Can you work these out from the model? Positions are in its coordinate system, mm. A direction names the side the tool comes from. Give positions to 0.01 mm unless a question says otherwise; leave off trailing zeros. Loops run counter-clockwise (first coordinate to the right, second up) from the corner with the lowest first, then second, coordinate; pieces in that order, holes last.
from build123d import *

# Parameters (mm, degrees)
BOSS_EXTRUDE1_DEPTH = 1.5
SKETCH2_R           = 3.38382201
BOSS_EXTRUDE2_DEPTH = 4.5
SKETCH3_R           = 2.5
CUT_EXTRUDE1_DEPTH  = 3
SKETCH4_R           = 1
CUT_EXTRUDE2_DEPTH  = 3.5
SKETCH5_R           = 0.55
CUT_EXTRUDE3_DEPTH  = 3.5
SCALE1_SCALE        = 2


with BuildPart() as part:
    # Sketch1 → Boss-Extrude1 (new body)
    with BuildSketch(Plane(origin=(0, 0, 0), x_dir=(1, 0, 0), z_dir=(0, 1, 0))):
        with BuildLine():
            Line((0.659413902, 3.335441996), (0, 3.4))
            ThreePointArc((0, 3.4), (-3.4, 0), (0, -3.4))
            Line((0, -3.4), (0.659413902, -3.335441996))
            Line((0.659413902, -3.335441996), (14.3, -2))
            ThreePointArc((14.3, -2), (16.3, 0), (14.3, 2))
            Line((14.3, 2), (0.659413902, 3.335441996))
        make_face()
    extrude(amount=BOSS_EXTRUDE1_DEPTH)

    # Sketch2 → Boss-Extrude2 (add)
    with BuildSketch(Plane.XZ):
        with Locations(Location((0, 0, 0), (0, 0, 270))):
            Circle(SKETCH2_R)
    extrude(amount=-BOSS_EXTRUDE2_DEPTH)

    # Sketch3 → Cut-Extrude1 (cut)
    with BuildSketch(Plane(origin=(0, 4.5, 0), x_dir=(1, 0, 0), z_dir=(0, 1, 0))):
        with Locations(Location((0, 0, 0), (0, 0, 270))):
            Circle(SKETCH3_R)
    extrude(amount=-CUT_EXTRUDE1_DEPTH, mode=Mode.SUBTRACT)

    # Sketch4 → Cut-Extrude2 (cut)
    with BuildSketch(Plane(origin=(0, 1.5, 0), x_dir=(1, 0, 0), z_dir=(0, 1, 0))):
        with Locations(Location((0, 0, 0), (0, 0, 270))):
            Circle(SKETCH4_R)
    extrude(amount=-CUT_EXTRUDE2_DEPTH, mode=Mode.SUBTRACT)

    # Sketch5 → Cut-Extrude3 (cut)
    with BuildSketch(Plane.XZ):
        with Locations(Location((14.3, 0, 0), (0, 0, 270))):
            Circle(SKETCH5_R)
        with Locations(Location((12.38, 0, 0), (0, 0, 270))):
            Circle(SKETCH5_R)
        with Locations(Location((10.46, 0, 0), (0, 0, 270))):
            Circle(SKETCH5_R)
        with Locations(Location((8.54, 0, 0), (0, 0, 270))):
            Circle(SKETCH5_R)
        with Locations(Location((6.62, 0, 0), (0, 0, 270))):
            Circle(SKETCH5_R)
        with Locations(Location((4.7, 0, 0), (0, 0, 270))):
            Circle(SKETCH5_R)
    extrude(amount=-CUT_EXTRUDE3_DEPTH, mode=Mode.SUBTRACT)


with BuildPart() as part_1:
    # Scale1: scaled about (4.137469707, 1.335828051, 0)
    add(part.part.scale(SCALE1_SCALE).moved(Location((-4.137469707, -1.335828051, 0))))


solid = part_1.part
(1) Suppose I cut it at D-D on y = 7. List the corners of the cut face in (x, z) for me.
Returned:
outline: circle Ø13.54 at (-4.14, 0); hole circle Ø10 at (-4.14, 0)
(2) Which directions (+Z, -Z, +X, -X, +Y, -Y) give clear straight access to the entire face, cutting with the end or side of a thin tool? Please do faces 5 (the cylindrical face through (15.7, 0.1, 0.2)), 6 (the flat face through (-4.1, 1.664, 2.2)).
Returned:
face 5: +Y, -Y
face 6: +Y
(3) Will these pins go through, and if not, where does the flat tip stop? P1, Ø2.5, axis at x = 24.46, z = 0, coming from the +Y side; P2, Ø2, axis at x = 22.5, y = 2.5, coming from the +Z side; P3, Ø1, axis at x = 14.5, y = -0.5, coming from the -Z side; P4, Ø2.5, axis at x = 20.62, z = 0, coming from the -Y side.
Returned:
P1: stops at y = 1.66
P2: stops at z = 4.25
P3: stops at z = -5.02
P4: stops at y = -1.34
(4) Suppose I cut it at A-A on y = -0.5. List the corners of the cut face in (x, z) for me, plus the area to 3 significant figures.
Returned:
outline: (-4.14, -6.8) - (24.46, -4) arc R4 ccw to (24.46, 4) - (-4.14, 6.8) arc R6.8 ccw to start; hole circle Ø4 at (-4.14, 0); hole circle Ø2.2 at (5.26, 0); hole circle Ø2.2 at (9.1, 0); hole circle Ø2.2 at (12.94, 0); hole circle Ø2.2 at (16.78, 0); hole circle Ø2.2 at (20.62, 0); hole circle Ø2.2 at (24.46, 0)
area: 371 mm2
(5) Please list where these lines run through material, in increasing order: probe 1 along Z at (x, y) = (-4, 5); probe 2 along Y at (x, z) = (26.5, -2.5); probe 3 along Z at (x, y) = (-8, 3).
Returned:
probe 1: z = -6.77 to -5, 5 to 6.77
probe 2: y = -1.34 to 1.66
probe 3: z = -5.56 to -3.18, 3.18 to 5.56
(6) Suppose I cut it at C-C on z = 0. Give the number of separate pieces and of enclosed holes in the cut face, plus the area to 3 significant figures.
Returned:
separate pieces: 8
enclosed holes: 0
area: 87.8 mm2
(7) Thinking about a two-plate mould opening in X: for faces 1 (the flat face through (8, -1.336, 1)), 2 (the cylindrical face through (28.46, 0.14, 0.09)), 3 (the cylindrical face through (25.553, 0.143, 0.143)), 4 (the cylindrical face through (-10.936, 0.143, -0.15)), which applies, pulls with the +X half, pulls with the -X half, needs draft (parallel to the pull), parting line crosses it, or undercut?
Returned:
face 1: needs draft
face 2: pulls with the +X half
face 3: undercut
face 4: pulls with the -X half
